For this review, take the finished solid that the model builds, in its own axes (mm). Round coordinates to 2 decimals unless told otherwise and drop trailing zeros. Order: outer loops, then holes, each group sorted by start corner. A loop starts at its lowest first (then second) coordinate and runs counter-clockwise, first axis right, second up. Notation, with made-up numbers: M -33,-20 L -16,-20 A11 cw -16,-13 Z; hole C 63,50.25 d3. An arc over 180 degrees is marked long. Use a Markdown table: item, result.
from build123d import *

# Parameters (mm, degrees)
F0_R     = 50
F0_R_2   = 28
F1_DEPTH = 38
F2_SIZE2 = 10
F2_SIZE  = 20
F3_R     = 10
F4_R     = 3


with BuildPart() as f1:
    # F0 (on Front) → F1 (new body)
    with BuildSketch(Plane.XZ):
        Circle(F0_R)
        Circle(F0_R_2, mode=Mode.SUBTRACT)
    extrude(amount=F1_DEPTH)

    # F2
    f2_edges = [f1.edges().sort_by_distance(p)[0] for p in [
        (-28, -38, 0),
    ]]
    f2_side = f1.faces().sort_by_distance((-28, -19, 0))[0]
    chamfer(f2_edges, length=F2_SIZE, length2=F2_SIZE2, reference=f2_side)

    # F3
    f3_edges = [f1.edges().sort_by_distance(p)[0] for p in [
        (-38, -38, 0),
    ]]
    fillet(f3_edges, radius=F3_R)

    # F4
    f4_edges = [f1.edges().sort_by_distance(p)[0] for p in [
        (-50, 0, 0),
        (-50, -38, 0),
    ]]
    fillet(f4_edges, radius=F4_R)


solid = f1.part
Q1. Add section D-D (y = -26.5). Write out the cut boundary in (x, z).
Determined:
| item | result |
|---|---|
| outline | C 0,0 d100; hole C 0,0 d64.5 |
Q2. Add section C-C (y = -8.5). Write out the cut boundary in (x, z), then the cut area to 3 significant figures.
Determined:
| item | result |
|---|---|
| outline | C 0,0 d100; hole C 0,0 d56 |
| area | 5,390 mm^2 |
Q3. Add section B-B (z = 0). Write out the cut boundary in (x, y), then the cut area to 3 significant figures.
Determined:
| item | result |
|---|---|
| outline | M -50,-35 A3 ccw -47,-38 L -44.18,-38 A10 ccw -35.24,-32.47 L -28,-18 L -28,0 L -47,0 A3 ccw -50,-3 Z; M 28,-18 L 35.24,-32.47 A10 ccw 44.18,-38 L 47,-38 A3 ccw 50,-35 L 50,-3 A3 ccw 47,0 L 28,0 Z |
| area | 1,450 mm^2 |
Q4. Wall thickness on line 1 along Z through (x, y) = (0, -9); line 2 along X through (y, z) = (-28.5, -24.5); line 3 along Z through (x, y) = (6.5, -27.5): over which ranges is each line inside the solid? List them lowest first. Write a range as [from, to].
Determined:
| item | result |
|---|---|
| line 1 | z = [-50, -28], [28, 50] |
| line 2 | x = [-43.59, -22.48], [22.48, 43.59] |
| line 3 | z = [-49.58, -32.1], [32.1, 49.58] |
Q5. Add section A-A (x = 0). Write out the cut boundary in (y, z), then the cut area to 3 significant figures.
Determined:
| item | result |
|---|---|
| outline | M -38,-47 A3 ccw -35,-50 L -3,-50 A3 ccw 0,-47 L 0,-28 L -18,-28 L -32.47,-35.24 A10 ccw -38,-44.18 Z; M -38,44.18 A10 ccw -32.47,35.24 L -18,28 L 0,28 L 0,47 A3 ccw -3,50 L -35,50 A3 ccw -38,47 Z |
| area | 1,450 mm^2 |
Q6. Clearance check with flat-ended pins moving along their axes: pin 1 (5 mm diameter, centred on x = 20, z = -32.5, fed in from -Y); pin 2 (4 mm diameter, centred on y = -5.5, z = 32.5, fed in from -X); pin 3 (10 mm diameter, centred on y = -12.5, z = -24, fed in from -X). State where each tip first meets the part, or that it passes through.
Determined:
| item | result |
|---|---|
| pin 1 | stops at y = -37.36 |
| pin 2 | stops at x = -39.62 |
| pin 3 | stops at x = -46.25 |
Q7. Draft analysis for pull direction Z (two halves, no side actions). For faces 1 (the cylindrical face through (47.69, -18.78, 15.02)), 2 (the flat face through (20, 0, -20)), 3 (the cylindrical face through (25.865, -8.874, -10.724)), state which applies: pulls with the +Z half, pulls with the -Z half, needs draft (parallel to the pull), parting line crosses it, or undercut.
Determined:
| item | result |
|---|---|
| face 1 | parting line crosses it |
| face 2 | needs draft |
| face 3 | undercut |
